Autodesk Inventor part; units mm, degrees
ref_plane "Start Plane" through (0, 0, 15) normal (0, 0, 1) x (1, 0, 0)
ref_plane "End Plane" through (0, 0, 179.8754) normal (0, 0, 1) x (1, 0, 0)
ref_plane "Work Plane4" through (299, -839, 15) normal (0, 0, -1) x (-1, 0, 0)
ref_plane "Start Plane" through (0, 0, 15) normal (0, 0, 1) x (1, 0, 0)
ref_plane "End Plane" through (0, 0, 179.8754) normal (0, 0, 1) x (1, 0, 0)
sketch "Sketch" plane through (0, 0, 0) normal (0, 0, 1) x (1, 0, 0)
  line L0 (-15, -9) -> (-15, 9)
  line L1 (-9, 15) -> (9, 15)
  line L2 (15, 9) -> (15, -9)
  line L3 (9, -15) -> (-9, -15)
  arc A0 (-15, -9) -> (-9, -15) centre (-9, -9) ccw
  arc A1 (-9, 15) -> (-15, 9) centre (-9, 9) ccw
  arc A2 (15, 9) -> (9, 15) centre (9, 9) ccw
  arc A3 (9, -15) -> (15, -9) centre (9, -9) ccw
  arc A4 (-9, 12) -> (-12, 9) centre (-9, 9) ccw
  line L4 (-9, 12) -> (9, 12)
  arc A5 (12, 9) -> (9, 12) centre (9, 9) ccw
  line L5 (12, 9) -> (12, -9)
  arc A6 (9, -12) -> (12, -9) centre (9, -9) ccw
  line L6 (9, -12) -> (-9, -12)
  arc A7 (-12, -9) -> (-9, -12) centre (-9, -9) ccw
  line L7 (-12, -9) -> (-12, 9)
  line L8 (0, 22.7397) -> (0, -22.7397) construction
  line L9 (-22.7397, 0) -> (22.7397, 0) construction
  dimension "d7" = 6
  dimension "d10" = 30
  dimension "d11" = 30
  dimension "d12" = 3
  dimension "d15" = 15
  dimension "d16" = 15
extrude "Body" add sketch "Sketch" along normal up to surface (164.8754 mm away) from surface at 15
sketch "Sketch3" plane through (0, 0, 0) normal (0, 0, 1) x (1, 0, 0)
  line L0 (0, 0) -> (10, 0)
ref_plane "Work Plane3" through (0, 0, 0) normal (0, -1, 0) x (1, 0, 0)
ref_plane "Work Plane4" through (299, -839, 15) normal (0, 0, -1) x (-1, 0, 0)
split "Split1" plane through (299, -839, 15) removes the side toward (0, 0, -1)
ref_plane "Work Plane5" through (9, 10, 188.8197) normal (0, -0.6667, 0.7454) x (1, 0, 0)
split "Split2" plane through (9, 10, 188.8197) removes the side toward (0, -0.6667, 0.7454)
ref_plane "Work Plane6" through (-9, -10, 188.8197) normal (0, 0.6667, 0.7454) x (1, 0, 0)
split "Split3" plane through (-9, -10, 188.8197) removes the side toward (0, 0.6667, 0.7454)
sketch "Sketch4" plane through (0, 0, 0) normal (0, -1, 0) x (1, 0, 0)
  line L0 (-2, 15) -> (12, 15)
  line L1 (-2, 179.8754) -> (12, 179.8754)
  dimension "d18" = 164.8754
equation "\"d7\" = G_IR"
equation "\"d10\" = G_H"
equation "\"d11\" = G_W"
equation "\"d12\" = G_T"
equation "\"d15\" = 0.5 * d10"
equation "\"d16\" = 0.5 * d11"
equation "\"d3\" = G_L"
equation "\"G_W\" = 30"
equation "\"G_H\" = 30"
equation "\"G_T\" = 3"
equation "\"G_IR\" = 6"
equation "\"G_L\" = d18"
equation "\"G_OFFSET_START\" = -15"
equation "\"G_OFFSET_END\" = -20.12461"
equation "\"d13\" = -G_OFFSET_START"
equation "\"d14\" = G_OFFSET_END + B_L"
properties part number "DIN EN 10219-2 - 30 x 30 x 3  - 164.88" material "Steel, Mild"
Check sheet for the modelled part. Datum: model origin and axes. Units: mm. A direction names the side the tool comes from. Round coordinates to 2 decimals unless told otherwise and drop trailing zeros. Loops run counter-clockwise (first coordinate to the right, second up) from the corner with the lowest first, then second, coordinate; pieces in that order, holes last. Notation, with made-up numbers: (-24, 20) -> (-13, 20) arc R24 cw to (-13, 56) -> close; hole circle Ø6 at (8, 4.25). An arc over 180 degrees is marked (long way). Answer in a Markdown table with one row per item.
Q1. Thickness scan on L1, parallel to Y at x = 0.5, z = 108.5; L2, parallel to Y at x = 10, z = 24. Record the ranges inside material, lowest first.
Data:
| item | result |
|---|---|
| L1 | y = -15 to -12, 12 to 15 |
| L2 | y = -14.92 to -11.83, 11.83 to 14.92 |
Q2. Sectioned sample at B-B on z = 31.5. Enter the section's corners in (x, y), then the cut area to 3 significant figures.
Data:
| item | result |
|---|---|
| outline | (-15, -9) arc R6 ccw to (-9, -15) -> (9, -15) arc R6 ccw to (15, -9) -> (15, 9) arc R6 ccw to (9, 15) -> (-9, 15) arc R6 ccw to (-15, 9) -> close; hole (-12, -9) arc R3 ccw to (-9, -12) -> (9, -12) arc R3 ccw to (12, -9) -> (12, 9) arc R3 ccw to (9, 12) -> (-9, 12) arc R3 ccw to (-12, 9) -> close |
| area | 301 mm^2 |
Q3. Go/stop test with a flat-tipped pin: P1, Ø6, axis at x = 7.5, y = -3, coming from the +Z side. Record where the tip stops, or that it passes through.
Data:
| item | result |
|---|---|
| P1 | passes through |
Q4. Release check for a two-part mould opening along Y. For faces 3 (the face through (11.14, -11.1, 92.32)), 4 (the face through (13.289, -13.196, 92.315)), 5 (the face through (-0.21, 12.395, 168.789)), 6 (the face through (-15, 0, 96)) record: released by +Y, released by -Y, zero draft, split by the parting line, or undercut.
Data:
| item | result |
|---|---|
| face 3 | undercut |
| face 4 | released by -Y |
| face 5 | released by +Y |
| face 6 | zero draft |
Q5. Sectioned sample at A-A on x = -4. Enter the section's corners in (y, z), then the cut area to 3 significant figures.
Data:
| item | result |
|---|---|
| outline | (-15, 15) -> (-12, 15) -> (-12, 169.14) -> (-15, 166.46) -> close; (12, 15) -> (15, 15) -> (15, 166.46) -> (12, 169.14) -> close |
| area | 917 mm^2 |
Q6. Sectioned sample at C-C on y = -3.75. Enter the section's corners in (x, z).
Data:
| item | result |
|---|---|
| outline | (-15, 15) -> (-12, 15) -> (-12, 176.52) -> (-15, 176.52) -> close; (12, 15) -> (15, 15) -> (15, 176.52) -> (12, 176.52) -> close |
Q7. Set-up check for faces 1 (the face through (12, 0, 96)), 2 (the face through (0, -15, 90)): record each of +Z, -Z, +X, -X, +Y, -Y from which the full face is reachable in a straight line by a thin tool's end or side.
Data:
| item | result |
|---|---|
| face 1 | +Z, -Z |
| face 2 | +Z, -Z, +X, -X, -Y |
